Drawing for the job (mm, zero at the part's lowest x, y, z). A direction names the side the tool comes from. Round coordinates to 2 decimals unless told otherwise and drop trailing zeros. Write each loop counter-clockwise with the first axis right and the second up, starting at its lowest first coordinate (ties: lowest second). Pieces come first, ordered by that corner, then holes. Notation, with made-up numbers: (32.5, 31) - (54.5, 31) arc R29 ccw to (54.5, 64) - close; hole circle Ø7 at (-22, 82.25). An arc over 180 degrees is marked (long way). One line per question, with ' | ' between items.
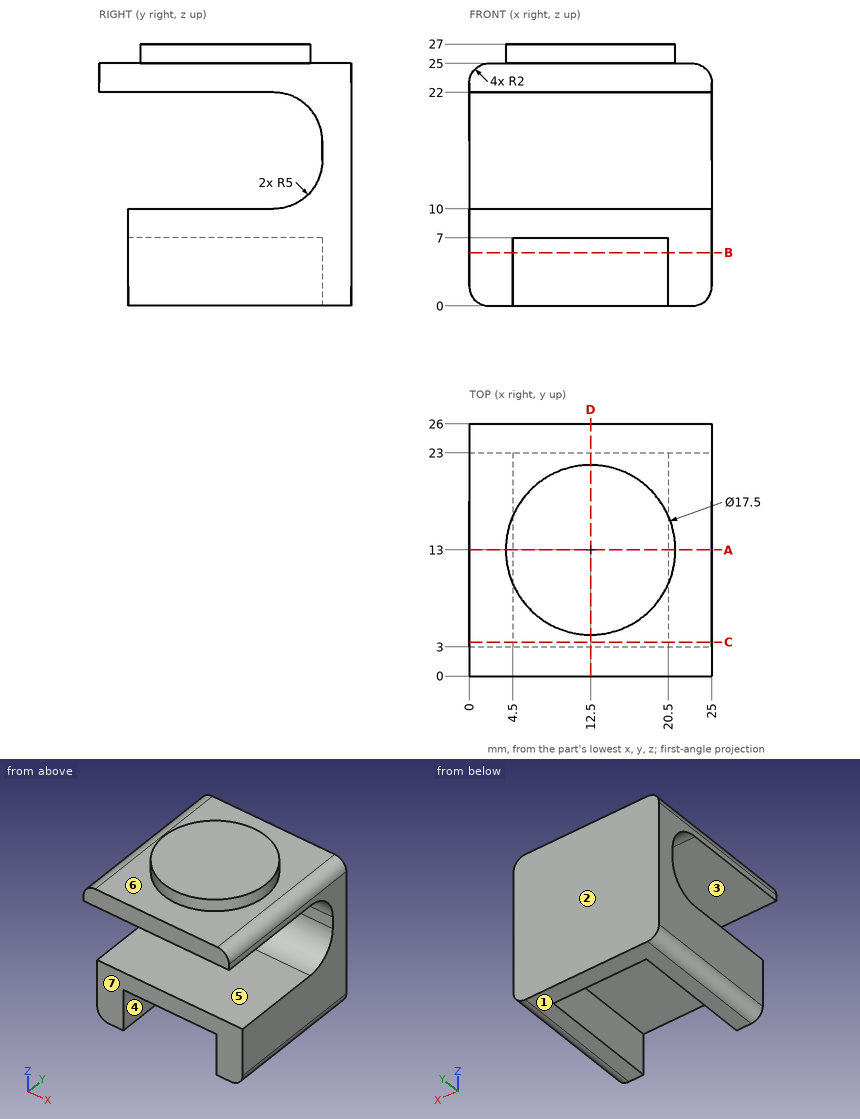
Q1. Drill centre lines: L1, parallel to Z at x = 6.25, y = 13.5; L2, parallel to X at y = 19.75, z = 6.75; L3, parallel to Y at x = 21.25, z = 9.75. Where is each one in solid material? Low to high. Write a range as from..to.
Found:
L1: 7..10, 22..27 | L2: 0..4.5, 20.5..25 | L3: 3..26
Q2. Which spindle directions (+Z, -Z, +X, -X, +Y, -Y) get a long thin tool onto all of the face, cutting with end or side? Do the marked faces 4, 5, 6 and 7. Say none if no direction does.
Found:
face 4: -Z, -Y | face 5: +X, -X, -Y | face 6: +Z | face 7: -Z, +X, -X, -Y
Q3. Saw through at A-A, the plane y = 13. List the corners of the cut face in (x, z), then the cut area to 3 significant figures.
Found:
outline: (0, 2) arc R2 ccw to (2, 0) - (4.5, 0) - (4.5, 7) - (20.5, 7) - (20.5, 0) - (23, 0) arc R2 ccw to (25, 2) - (25, 10) - (0, 10) - close; (0, 22) - (25, 22) - (25, 23) arc R2 ccw to (23, 25) - (21.25, 25) - (21.25, 27) - (3.75, 27) - (3.75, 25) - (2, 25) arc R2 ccw to (0, 23) - close | area: 245 mm^2
Q4. Drop flat-ended pins along their axis: pin 1 (3.5 mm diameter, centred on x = 11.5, z = 2, fed in from -Y); pin 2 (6 mm diameter, centred on x = 21, y = 3.5, fed in from +Z); pin 3 (8 mm diameter, centred on x = 6.5, z = 5.5, fed in from -Y). Give the stop position or say it passes through.
Found:
pin 1: y = 23 | pin 2: z = 25 | pin 3: y = 3
Q5. Pull direction Z, two halves, no side cores. Call the marked faces 1, 2 and 3: +Z half, -Z half, draft (parallel to the pull), parting line (faces both ways), or undercut.
Found:
face 1: -Z half | face 2: draft | face 3: undercut
Q6. Saw through at D-D, the plane x = 12.5. List the corners of the cut face in (y, z).
Found:
outline: (0, 22) - (18, 22) arc R5 cw to (23, 17) - (23, 15) arc R5 cw to (18, 10) - (3, 10) - (3, 7) - (23, 7) - (23, 0) - (26, 0) - (26, 25) - (21.75, 25) - (21.75, 27) - (4.25, 27) - (4.25, 25) - (0, 25) - close
Q7. Saw through at B-B, the plane z = 5.5. List the corners of the cut face in (x, y).
Found:
outline: (0, 3) - (4.5, 3) - (4.5, 23) - (20.5, 23) - (20.5, 3) - (25, 3) - (25, 26) - (0, 26) - close
Q8. Saw through at C-C, the plane y = 3.5. List the corners of the cut face in (x, z), then the cut area to 3 significant figures.
Found:
outline: (0, 2) arc R2 ccw to (2, 0) - (4.5, 0) - (4.5, 7) - (20.5, 7) - (20.5, 0) - (23, 0) arc R2 ccw to (25, 2) - (25, 10) - (0, 10) - close; (0, 22) - (25, 22) - (25, 23) arc R2 ccw to (23, 25) - (2, 25) arc R2 ccw to (0, 23) - close | area: 210 mm^2
